Build history of the part. All positions in model axes, mm. Coordinates: 2 decimals unless noted, no trailing zeros. Loops run counter-clockwise (first coordinate to the right, second up) from the corner with the lowest first, then second, coordinate; pieces in that order, holes last.
(1) Flat gauge pins, fed straight in: P1, Ø0.9, axis at x = 24.5, z = -1, coming from the +Y side; P2, Ø4, axis at x = 15, y = 193, coming from the -Z side; P3, Ø1.5, axis at x = 18, z = -2, coming from the -Y side; P4, Ø0.9, axis at y = 11.5, z = -1, coming from the -X side. Where does each tip first touch, or does it go through?
(2) Two-plate mould, pull along X, no slides. Class faces 1 (the face through (14.28, 189.78, -1.48)), 2 (the face through (96, 122, 0)): pulls with the +X half, pulls with the -X half, needs draft (parallel to the pull), parting line crosses it, or undercut.
(3) Wall check: L1, parallel to X at y = 225, z = -1.7; L2, parallel to Y at x = 15, z = -2.35; L3, parallel to Y at x = 44, z = -1.5. Give the ranges that are in metal, low to high.
(4) Slice it at D-D (y = 193). Give the cut face in (x, z), and give its area (3 significant figures).
(5) Slice it at A-A (x = 139). Give the cut face in (y, z), and give its area (3 significant figures).
(6) Slice it at C-C (z = -2). Give the number of separate pieces and of enclosed holes in the cut face, and give its area (3 significant figures).
(7) Slice it at B-B (y = 225). Give the cut face in (x, z).
from build123d import *

# Parameters (mm, degrees)
BASE_FLANGE1_DEPTH = 3
CHAMFER1_SIZE      = 2
SKETCH3_R          = 3
CUT_EXTRUDE1_DEPTH = 10
SKETCH4_R          = 3.3
SKETCH4_R_2        = 7.5
CUT_EXTRUDE2_DEPTH = 10


# Sheet-metal steps are written as plain solids
with BuildPart() as part:
    # Sketch1 → Base-Flange1 (new body)
    with BuildSketch(Plane.XY):
        Polygon((0, 208), (32, 208), (32, 240), (190, 240), (190, 32), (158, 32), (158, 0), (32, 0), (32, 32), (0, 32), align=None)
    extrude(amount=-BASE_FLANGE1_DEPTH)

    # Chamfer1
    chamfer1_edges = [part.edges().sort_by_distance(p)[0] for p in [
        (190, 32, -1.5),
        (158, 0, -1.5),
        (32, 0, -1.5),
        (0, 32, -1.5),
        (0, 208, -1.5),
        (32, 240, -1.5),
        (190, 240, -1.5),
    ]]
    chamfer(chamfer1_edges, length=CHAMFER1_SIZE)

    # Sketch3 → Cut-Extrude1 (cut)
    with BuildSketch(Plane.XY):
        with Locations((130.5, 215)):
            Circle(SKETCH3_R)
        with Locations((173.5, 215)):
            Circle(SKETCH3_R)
    extrude(amount=-CUT_EXTRUDE1_DEPTH, mode=Mode.SUBTRACT)

    # Sketch4 → Cut-Extrude2 (cut)
    with BuildSketch(Plane.XY):
        with Locations((42, 225)):
            Circle(SKETCH4_R)
        with Locations((120, 225)):
            Circle(SKETCH4_R)
        with Locations((175, 193)):
            Circle(SKETCH4_R)
        with Locations((175, 135)):
            Circle(SKETCH4_R)
        with Locations((175, 44)):
            Circle(SKETCH4_R)
        with Locations((139, 15)):
            Circle(SKETCH4_R)
        with Locations((44, 15)):
            Circle(SKETCH4_R)
        with Locations((15, 193)):
            Circle(SKETCH4_R)
        with Locations((15, 47)):
            Circle(SKETCH4_R)
        with Locations((152, 215)):
            Circle(SKETCH4_R_2)
    extrude(amount=-CUT_EXTRUDE2_DEPTH, mode=Mode.SUBTRACT)


solid = part.part
Response values:
1. P1: stops at y = 208
1. P2: passes through
1. P3: stops at y = 32
1. P4: stops at x = 32
2. face 1: undercut
2. face 2: needs draft
3. L1: x = 32 to 38.7, 45.3 to 116.7, 123.3 to 190
3. L2: y = 32 to 43.7, 50.3 to 189.7, 196.3 to 208
3. L3: y = 0 to 11.7, 18.3 to 222.38, 227.62 to 240
4. outline: (0, -3) - (11.7, -3) - (11.7, 0) - (0, 0) - close; (18.3, -3) - (171.7, -3) - (171.7, 0) - (18.3, 0) - close; (178.3, -3) - (190, -3) - (190, 0) - (178.3, 0) - close
4. area: 530 mm2
5. outline: (0, -3) - (11.7, -3) - (11.7, 0) - (0, 0) - close; (18.3, -3) - (240, -3) - (240, 0) - (18.3, 0) - close
5. area: 700 mm2
6. separate pieces: 1
6. enclosed holes: 12
6. area: 42,000 mm2
7. outline: (32, -3) - (38.7, -3) - (38.7, 0) - (32, 0) - close; (45.3, -3) - (116.7, -3) - (116.7, 0) - (45.3, 0) - close; (123.3, -3) - (190, -3) - (190, 0) - (123.3, 0) - close
